Could you check a few things on this model? Use its own coordinates, in mm. A direction names the side the tool comes from. Round coordinates to 2 decimals unless told otherwise and drop trailing zeros. Loops run counter-clockwise (first coordinate to the right, second up) from the corner with the lowest first, then second, coordinate; pieces in that order, holes last. Notation, with made-up numbers: (-38.75, 33.25) -> (-5.75, 33.25) arc R30 cw to (-5.75, 62.25) -> close; hole circle Ø10 at (26.5, 70). An arc over 180 degrees is marked (long way). One line per item, written item: value.
Autodesk Inventor part; units mm, degrees
ref_plane "YZ Plane" through (0, 0, 0) normal (1, 0, 0) x (0, 1, 0)
ref_plane "XZ Plane" through (0, 0, 0) normal (0, 1, 0) x (-1, 0, 0)
ref_plane "XY Plane" through (0, 0, 0) normal (0, 0, 1) x (1, 0, 0)
sketch "Náčrt11" plane through (0, 0, 0) normal (1, 0, 0) x (0, 1, 0)
  line L0 (-6.6, 0) -> (39.6, 0)
  line L1 (0, -240) -> (0, 40)
  line L2 (0, 0) -> (33, 0)
  line L3 (33, 0) -> (33, -10)
  line L4 (33, -10) -> (0, -10)
  line L5 (0, -10) -> (0, 0)
  line L6 (0, -10) -> (7.5, -10)
  line L7 (7.5, -10) -> (7.5, -200)
  line L8 (7.5, -200) -> (0, -200)
  line L9 (0, -200) -> (0, -10)
  point P0 (33, 0)
  point P1 (0, -200)
  dimension "d109" = 33
  dimension "d110" = 10
  dimension "d111" = 7.5
  dimension "d112" = 190
revolve "Rotace2" add sketch "Náčrt11" angle 360 about axis through (0, 0, -10) along (0, 0, 1)
sketch "Náčrt12" plane through (0, 0, -10) normal (0, 0, -1) x (-1, 0, 0)
  line L0 (46.2, 0) -> (-46.2, 0)
  line L1 (0, -46.2) -> (0, 46.2)
  circle A0 centre (0, 0) radius 25 construction
  point P0 (0, 25)
  point P1 (-25, 0)
  point P2 (25, 0)
  point P3 (0, -25)
  dimension "d114" = 50
hole "Díra4" at (0, 25, -10) at (25, 0, -10) at (-25, 0, -10) at (0, -25, -10) direction (0, 0, 1) diameter 6.6 end through all counterbore diameter 11.4 counterbore depth 6.5
chamfer "Zkosení4" distance 10 distance2 7.5 1 edges at (0, -7.5, -200) measured on face at (0.6035, 7.4757, -136.6667)
fillet "Zaoblení12" radius 1 1 edges at (0, -33, -10)
fillet "Zaoblení13" radius 10 1 edges at (0, -7.5, -10)
properties part number "Drzak_kamera"
(1) Thinking about a two-plate mould opening in X: for faces 3 (the face through (0, 0, 0)), 4 (the face through (0.33, -7.493, -106.19)), 5 (the face through (-21.78, -0.72, -1.73)), which applies, released by +X, released by -X, zero draft, split by the parting line, or undercut?
Recorded:
face 3: zero draft
face 4: split by the parting line
face 5: undercut
(2) I'm going to push flat-ended pins straight in: pin 1 Ø5.5 at (x, y) = (0, 25) entering from +Z; pin 2 Ø12.5 at (x, y) = (0, 23.5) entering from -Z; pin 3 Ø18 at (x, y) = (-25, 0) entering from -Z; pin 4 Ø9 at (x, y) = (25, 0) entering from -Z. Where does each tip first touch, or does it pass through?
Recorded:
pin 1: through
pin 2: z = -10
pin 3: z = -10.11
pin 4: z = -3.5
(3) If I drill on L1, parallel to Y at x = 0, z = -2; L2, parallel to X at y = 0, z = -6, over which ranges is the centre line in solid material (lowest first)?
Recorded:
L1: -33 to -28.3, -21.7 to 21.7, 28.3 to 33
L2: -33 to -30.7, -19.3 to 19.3, 30.7 to 33
(4) For faces 1 (the face through (2.5, -22.5, -3.5)), 2 (the face through (-12.6, 30.5, -4.6)), which set-ups out of +Z, -Z, +X, -X, +Y, -Y let a thin tool reach every point of the face, with its end or its side?
Recorded:
face 1: -Z
face 2: +Z, -Z
(5) If we section it at A-A, the plane z = -185.5: Please give me the cut outline in (x, y).
Recorded:
outline: circle Ø15 at (0, 0)
